For this review, take the finished solid that the model builds, in its own axes (mm). A direction names the side the tool comes from. Round coordinates to 2 decimals unless told otherwise and drop trailing zeros. Write each loop counter-clockwise with the first axis right and the second up, starting at its lowest first coordinate (ties: lowest second). Pieces come first, ordered by that corner, then holes. Notation, with made-up numbers: (70.25, -24.75) -> (116.25, -24.75) arc R17 cw to (116.25, 0.25) -> close; hole circle Ø3 at (60.25, 77.5). An arc over 180 degrees is marked (long way). Answer in a Markdown table with one row per item.
from build123d import *

# Parameters (mm, degrees)
ESQUISSE1_R      = 8
EXTRUSION1_DEPTH = 1
ESQUISSE2_R      = 6.1
EXTRUSION2_DEPTH = 8
ESQUISSE3_R      = 8
EXTRUSION3_DEPTH = 7
ESQUISSE4_R      = 2
EXTRUSION4_DEPTH = 20.595917942


with BuildPart() as part:
    # Esquisse1 → Extrusion1 (new body)
    with BuildSketch(Plane(origin=(0, 0, 0), x_dir=(1, 0, 0), z_dir=(0, 1, 0))):
        with Locations(Location((0, 0, 0), (0, 0, 270))):
            Circle(ESQUISSE1_R)
    extrude(amount=EXTRUSION1_DEPTH)

    # Esquisse2 → Extrusion2 (add)
    with BuildSketch(Plane(origin=(0, 1, 0), x_dir=(-1, 0, 0), z_dir=(0, 1, 0))):
        with Locations(Location((0, 0, 0), (0, 0, 90))):
            Circle(ESQUISSE2_R)
    extrude(amount=EXTRUSION2_DEPTH)

    # Esquisse3 → Extrusion3 (add)
    with BuildSketch(Plane(origin=(0, 9, 0), x_dir=(-1, 0, 0), z_dir=(0, 1, 0))):
        with Locations(Location((0, 0, 0), (0, 0, 90))):
            Circle(ESQUISSE3_R)
    extrude(amount=EXTRUSION3_DEPTH)

    # Esquisse4 → Extrusion4 (cut, through all)
    with BuildSketch(Plane(origin=(0, 16, 0), x_dir=(-1, 0, 0), z_dir=(0, 1, 0))):
        with Locations(Location((0, 0, 0), (0, 0, 90))):
            Circle(ESQUISSE4_R)
    extrude(amount=-EXTRUSION4_DEPTH, mode=Mode.SUBTRACT)


solid = part.part
1) Consider section A-A on z = 0. State the section outline as (x, y) points, then the cut area to 3 significant figures.
Solved:
| item | result |
|---|---|
| outline | (-8, 0) -> (-2, 0) -> (-2, 16) -> (-8, 16) -> (-8, 9) -> (-6.1, 9) -> (-6.1, 1) -> (-8, 1) -> close; (2, 0) -> (8, 0) -> (8, 1) -> (6.1, 1) -> (6.1, 9) -> (8, 9) -> (8, 16) -> (2, 16) -> close |
| area | 162 mm² |
2) For line 1 (Y direction, x = -3.25, z = -5.75); line 2 (X direction, y = 9.5, z = 0); line 3 (X direction, y = 4.75, z = 0), list the stretches that pass through material, from the lowest coordinate up. Write a range as [from, to].
Solved:
| item | result |
|---|---|
| line 1 | [0, 1], [9, 16] |
| line 2 | [-8, -2], [2, 8] |
| line 3 | [-6.1, -2], [2, 6.1] |
3) For faces 1 (the flat face through (-6, 1, -2)), 2 (the flat face through (-2, 0, 2)), list the 3-axis set-ups (+Z, -Z, +X, -X, +Y, -Y) from which the entire face can be reached by the end or side of a thin tool; tool diameter is ignored.
Solved:
| item | result |
|---|---|
| face 1 | none |
| face 2 | +Z, -Z, +X, -X, -Y |
4) Consider section B-B on x = 0. State the section outline as (y, z) points.
Solved:
| item | result |
|---|---|
| outline | (0, -8) -> (1, -8) -> (1, -6.1) -> (9, -6.1) -> (9, -8) -> (16, -8) -> (16, -2) -> (0, -2) -> close; (0, 2) -> (16, 2) -> (16, 8) -> (9, 8) -> (9, 6.1) -> (1, 6.1) -> (1, 8) -> (0, 8) -> close |
5) Mouldability with a two-part tool opening along Z and no side actions: class faces 3 (the cylindrical face through (-2, 8, 0)), 4 (the cylindrical face through (-7.81, 0.49, -1.73)), 5 (the flat face through (-6, 9, -2)) as pulls with the +Z half, pulls with the -Z half, needs draft (parallel to the pull), parting line crosses it, or undercut.
Solved:
| item | result |
|---|---|
| face 3 | undercut |
| face 4 | parting line crosses it |
| face 5 | needs draft |
6) Consider section D-D on x = -2.5. State the section outline as (y, z) points, then the cut area to 3 significant figures.
Solved:
| item | result |
|---|---|
| outline | (0, -7.6) -> (1, -7.6) -> (1, -5.56) -> (9, -5.56) -> (9, -7.6) -> (16, -7.6) -> (16, 7.6) -> (9, 7.6) -> (9, 5.56) -> (1, 5.56) -> (1, 7.6) -> (0, 7.6) -> close |
| area | 211 mm² |
7) Clearance check with flat-ended pins moving along their axes: pin 1 Ø4 at (y, z) = (4, -6) entering from +X; pin 2 Ø2 at (x, y) = (-4, 9) entering from +Z; pin 3 Ø2 at (x, z) = (-0.5, 1.5) entering from -Y. State where each tip first meets the part, or that it passes through.
Solved:
| item | result |
|---|---|
| pin 1 | x = 4.61 |
| pin 2 | z = 7.42 |
| pin 3 | y = 0 |
8) Consider section C-C on y = 5.5. State the section outline as (x, z) points, then the cut area to 3 significant figures.
Solved:
| item | result |
|---|---|
| outline | circle Ø12.2 at (0, 0); hole circle Ø4 at (0, 0) |
| area | 104 mm² |
